Could you check a few things on this model? Use its own coordinates, in mm. A direction names the side the tool comes from. Give positions to 0.01 mm unless a question says otherwise; leave off trailing zeros. Write each loop counter-clockwise with the first axis right and the second up, starting at its lowest first coordinate (ties: lowest second). Pieces come first, ordered by that corner, then holes. Notation, with made-up numbers: (-19.5, -39.75) -> (2.5, -39.75) arc R11 cw to (2.5, -28.75) -> close; hole circle Ø5 at (31, 16.25). An arc over 180 degrees is marked (long way). One line per question, with ' | ' between items.
from build123d import *

# Parameters (mm, degrees)
SKETCH1_R           = 32
SKETCH1_R_2         = 6
BOSS_EXTRUDE1_DEPTH = 0.3


with BuildPart() as part:
    # Sketch1 → Boss-Extrude1 (new body)
    with BuildSketch(Plane(origin=(0, 0, 0), x_dir=(1, 0, 0), z_dir=(0, 1, 0))):
        Circle(SKETCH1_R)
        Circle(SKETCH1_R_2, mode=Mode.SUBTRACT)
        with BuildLine():
            ThreePointArc((27, 0), (4.688500797, 26.589809331), (-25.371700761, 9.23454387))
            ThreePointArc((-25.371700761, 9.23454387), (-25.072864522, 8.593687488), (-24.43200814, 8.892523726))
            ThreePointArc((-24.43200814, 8.892523726), (4.514852619, 25.605001578), (26, 0))
            ThreePointArc((26, 0), (26.5, -0.5), (27, 0))
        make_face(mode=Mode.SUBTRACT)
        with BuildLine():
            ThreePointArc((0, 21.5), (-21.17336669, 3.73343582), (-7.353433082, -20.203391347))
            ThreePointArc((-7.353433082, -20.203391347), (-6.712576699, -19.904555108), (-7.011412938, -19.263698726))
            ThreePointArc((-7.011412938, -19.263698726), (-20.188558937, 3.559787642), (0, 20.5))
            ThreePointArc((0, 20.5), (0.5, 21), (0, 21.5))
        make_face(mode=Mode.SUBTRACT)
        with BuildLine():
            ThreePointArc((16, 0), (2.778370843, 15.756924048), (-15.035081933, 5.472322293))
            ThreePointArc((-15.035081933, 5.472322293), (-14.736245694, 4.831465911), (-14.095389312, 5.13030215))
            ThreePointArc((-14.095389312, 5.13030215), (2.604722665, 14.772116295), (15, 0))
            ThreePointArc((15, 0), (15.5, -0.5), (16, 0))
        make_face(mode=Mode.SUBTRACT)
        with BuildLine():
            ThreePointArc((0, -21.5), (21.17336669, -3.73343582), (7.353433082, 20.203391347))
            ThreePointArc((7.353433082, 20.203391347), (6.712576699, 19.904555108), (7.011412938, 19.263698726))
            ThreePointArc((7.011412938, 19.263698726), (20.188558937, -3.559787642), (0, -20.5))
            ThreePointArc((0, -20.5), (-0.5, -21), (0, -21.5))
        make_face(mode=Mode.SUBTRACT)
        with BuildLine():
            ThreePointArc((0, 10.5), (-10.340481407, 1.823305866), (-3.591211505, -9.866772518))
            ThreePointArc((-3.591211505, -9.866772518), (-2.950355123, -9.56793628), (-3.249191362, -8.927079897))
            ThreePointArc((-3.249191362, -8.927079897), (-9.355673654, 1.649657688), (0, 9.5))
            ThreePointArc((0, 9.5), (0.5, 10), (0, 10.5))
        make_face(mode=Mode.SUBTRACT)
        with BuildLine():
            ThreePointArc((0, -10.5), (10.340481407, -1.823305866), (3.591211505, 9.866772518))
            ThreePointArc((3.591211505, 9.866772518), (2.950355123, 9.56793628), (3.249191362, 8.927079897))
            ThreePointArc((3.249191362, 8.927079897), (9.355673654, -1.649657688), (0, -9.5))
            ThreePointArc((0, -9.5), (-0.5, -10), (0, -10.5))
        make_face(mode=Mode.SUBTRACT)
        with BuildLine():
            ThreePointArc((-16, 0), (-2.778370843, -15.756924048), (15.035081933, -5.472322293))
            ThreePointArc((15.035081933, -5.472322293), (14.736245694, -4.831465911), (14.095389312, -5.13030215))
            ThreePointArc((14.095389312, -5.13030215), (-2.604722665, -14.772116295), (-15, 0))
            ThreePointArc((-15, 0), (-15.5, 0.5), (-16, 0))
        make_face(mode=Mode.SUBTRACT)
        with BuildLine():
            ThreePointArc((-27, 0), (-4.688500797, -26.589809331), (25.371700761, -9.23454387))
            ThreePointArc((25.371700761, -9.23454387), (25.072864522, -8.593687488), (24.43200814, -8.892523726))
            ThreePointArc((24.43200814, -8.892523726), (-4.514852619, -25.605001578), (-26, 0))
            ThreePointArc((-26, 0), (-26.5, 0.5), (-27, 0))
        make_face(mode=Mode.SUBTRACT)
    extrude(amount=BOSS_EXTRUDE1_DEPTH)


solid = part.part
Q1. Imagine slicing it at C-C on z = 28.5. Please give me the cut outline in (x, y).
Answer below:
outline: (-14.55, 0) -> (14.55, 0) -> (14.55, 0.3) -> (-14.55, 0.3) -> close
Q2. Imagine slicing it at B-B on y = 0.2. Count the separate pieces of the cut face and the enclosed holes in it, and give its area (3 significant figures).
Answer below:
separate pieces: 1 | enclosed holes: 9 | area: 2,690 mm^2
Q3. If I drill on line 1 along Z through (x, y) = (23, 0.1); line 2 along X through (y, z) = (0.15, -18); line 3 along X through (y, z) = (0.25, 28.5), over which ranges is the centre line in solid material (lowest first)?
Answer below:
line 1: z = -22.25 to -14.14, -12.12 to 12.12, 14.14 to 22.25 | line 2: x = -26.46 to -20.12, -18.76 to -11.76, -9.81 to 9.81, 11.76 to 18.76, 20.12 to 26.46 | line 3: x = -14.55 to 14.55
Q4. On a 3-axis mill with a long thin cutter (end or side, diameter ignored), from which of +Z, -Z, +X, -X, +Y, -Y can I reach the whole of each face in a straight line? I mean faces 1 (the flat face through (7, 0.3, 0)), 2 (the cylindrical face through (10.3, 0.15, 2.03)). Say none if no direction works.
Answer below:
face 1: +Z, -Z, +X, -X, +Y | face 2: +Y, -Y
Q5. Imagine slicing it at A-A on x = -22.5. Please give me the cut outline in (y, z).
Answer below:
outline: (0, -22.75) -> (0.3, -22.75) -> (0.3, -14.92) -> (0, -14.92) -> close; (0, -13.03) -> (0.3, -13.03) -> (0.3, 13.03) -> (0, 13.03) -> close; (0, 14.92) -> (0.3, 14.92) -> (0.3, 22.75) -> (0, 22.75) -> close
Q6. If we mould it in two halves opening along Z, with no side actions, what happens to faces 3 (the flat face through (7, 0, 0)), 4 (the cylindrical face through (2.32, 0.15, -14.82)), 5 (the cylindrical face through (4.01, 0.15, -25.69))? For each: +Z half, -Z half, draft (parallel to the pull), parting line (faces both ways), or undercut.
Answer below:
face 3: draft | face 4: undercut | face 5: undercut
